Work out the finished part from the listing and answer in its coordinate system (mm). Face numbers are marked on the shaded views. A direction names the side the tool comes from. Round coordinates to 2 decimals unless told otherwise and drop trailing zeros. Write each loop counter-clockwise with the first axis right and the second up, starting at its lowest first coordinate (ties: lowest second). Pieces come first, ordered by that corner, then holes. Notation, with made-up numbers: (82, 27) - (87, 27) arc R4 ccw to (87, 34) - close; hole circle Ø5 at (12, -26.75). An arc over 180 degrees is marked (long way). Write item = value, one per line. Start each with the question number.
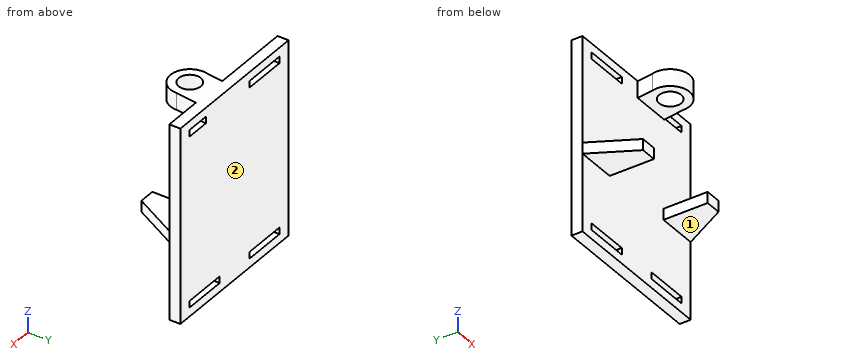
from build123d import *

# Parameters (mm, degrees)
SKETCH1_W               = 45.466
SKETCH1_H               = 55.88
SKETCH1_W_2             = 12.7
SKETCH1_H_2             = 1.905
BOSS_EXTRUDE1_DEPTH     = 3.175
BOSS_EXTRUDE2_DEPTH     = 3.175
BOSS_EXTRUDE3_START     = -4.826
BOSS_EXTRUDE3_OUTLINE_R = 3.175
BOSS_EXTRUDE3_DEPTH     = 4.826


# Read off the part's stored shape, not the designer's step: Boss-Extrude3
with BuildPart() as part:
    # Sketch1 → Boss-Extrude1 (new body)
    with BuildSketch(Plane(origin=(0, 0, 0), x_dir=(1, 0, 0), z_dir=(0, 1, 0))):
        with Locations((22.733, 27.94)):
            Rectangle(SKETCH1_W, SKETCH1_H)
        with Locations((35.306, 52.3875)):
            Rectangle(SKETCH1_W_2, SKETCH1_H_2, mode=Mode.SUBTRACT)
        with Locations((10.16, 52.3875)):
            Rectangle(SKETCH1_W_2, SKETCH1_H_2, mode=Mode.SUBTRACT)
        with Locations((35.306, 3.4925)):
            Rectangle(SKETCH1_W_2, SKETCH1_H_2, mode=Mode.SUBTRACT)
        with Locations((10.16, 3.4925)):
            Rectangle(SKETCH1_W_2, SKETCH1_H_2, mode=Mode.SUBTRACT)
    extrude(amount=BOSS_EXTRUDE1_DEPTH)

    # 3DSketch2 → Boss-Extrude2 (add)
    with BuildSketch(Plane(origin=(34.036, 0, -30.48), x_dir=(-1, 0, 0), z_dir=(0, 0, 1))):
        Polygon((0, 0), (0, 12.7), (-4.572, 12.7), (-11.43, 0), align=None)
        Polygon((22.606, 0), (22.606, 12.7), (27.178, 12.7), (34.036, 0), align=None)
    extrude(amount=-BOSS_EXTRUDE2_DEPTH)

    # Boss-Extrude3 outline → Boss-Extrude3 (add)
    with BuildSketch(Plane.XY.offset(BOSS_EXTRUDE3_START)):
        with BuildLine():
            Line((23.215006065, 0), (22.584264524, -4.606399832))
            ThreePointArc((22.584264524, -4.606399832), (27.182231525, -11.604883936), (33.49225, -6.1))
            Line((33.49225, -6.1), (34.76225, 3.175))
            Line((34.76225, 3.175), (28.956, 3.175))
            Line((28.956, 3.175), (28.956, 0))
            Line((28.956, 0), (23.215006065, 0))
        make_face()
        with Locations((27.936, -6.1)):
            Circle(BOSS_EXTRUDE3_OUTLINE_R, mode=Mode.SUBTRACT)
    extrude(amount=BOSS_EXTRUDE3_DEPTH)


solid = part.part
1. Which of the six approach directions +Z, -Z, +X, -X, +Y, -Y give full straight-line access (tool end or side, diameter ignored) to the marked faces 1 and 2?
2. Find section D-D on y = -1.75. Give the vertices of the cut face in (x, z) (3 decimals).
3. Find section B-B on x = 32.5. Give the vertices of the cut face in (y, z) (3 decimals).
4. Each of these flat-tipped pins is pushed along its axis until it touches: pin 1 (1.6 mm diameter, centred on y = -7, z = -31.5, fed in from +X); pin 2 (1.6 mm diameter, centred on y = -3, z = -32, fed in from -X); pin 3 (5.5 mm diameter, centred on x = 8.5, y = -5.5, fed in from +Z). Where does it stop, or does it pass through?
5. Consider line 1 (Z direction, x = 15.5, y = 1.75) (3 decimals); line 2 (Z direction, x = 30, y = 1) (3 decimals); line 3 (X direction, y = -7.5, z = -31.5). Determine where each line is inside the solid, lowest interval first.
6. Find section C-C on x = 39.5. Give the vertices of the cut face in (y, z) (3 decimals).
7. Find section A-A on y = -7.25. Give the vertices of the cut face in (x, z) (3 decimals), plus the area to 3 significant figures.
Answer key:
q1.face_1 = -Z, +X, -X, -Y
q1.face_2 = +Z, -Z, +X, -X, +Y
q2.outline = (0.945, -33.655) - (11.43, -33.655) - (11.43, -30.48) - (0.945, -30.48) - close; (22.975, -4.826) - (34.088, -4.826) - (34.088, 0) - (22.975, 0) - close; (34.036, -33.655) - (44.521, -33.655) - (44.521, -30.48) - (34.036, -30.48) - close
q3.outline = (-9.269, -4.826) - (0, -4.826) - (0, -51.435) - (3.175, -51.435) - (3.175, 0) - (-9.269, 0) - close; (0, -55.88) - (3.175, -55.88) - (3.175, -53.34) - (0, -53.34) - close
q4.pin_1 = 42.12
q4.pin_2 = 1.19
q4.pin_3 = -30.48
q5.line_1 = -55.88 to -53.34, -51.435 to -4.445, -2.54 to 0
q5.line_2 = -55.88 to -53.34, -51.435 to 0
q5.line_3 = 4.05 to 11.43, 34.04 to 41.42
q6.outline = (-11.048, -33.655) - (0, -33.655) - (0, -51.435) - (3.175, -51.435) - (3.175, -4.445) - (0, -4.445) - (0, -30.48) - (-11.048, -30.48) - close; (0, -55.88) - (3.175, -55.88) - (3.175, -53.34) - (0, -53.34) - close; (0, -2.54) - (3.175, -2.54) - (3.175, 0) - (0, 0) - close
q7.outline = (3.915, -33.655) - (11.43, -33.655) - (11.43, -30.48) - (3.915, -30.48) - close; (22.5, -4.826) - (24.977, -4.826) - (24.977, 0) - (22.5, 0) - close; (30.895, -4.826) - (33.372, -4.826) - (33.372, 0) - (30.895, 0) - close; (34.036, -33.655) - (41.551, -33.655) - (41.551, -30.48) - (34.036, -30.48) - close
q7.area = 71.6 mm²
